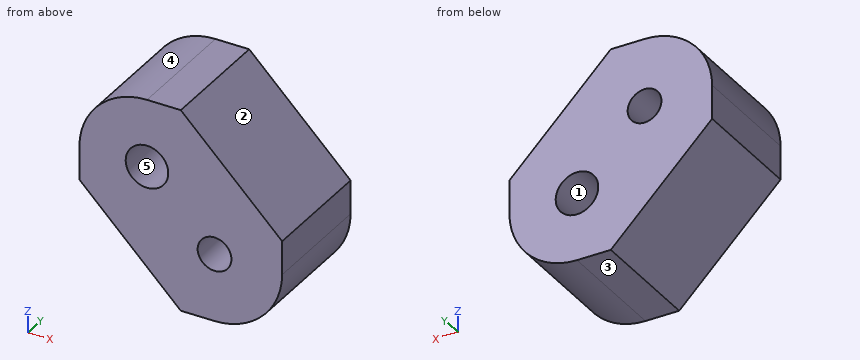
```python
from build123d import *

# Parameters (mm, degrees)
SKETCH1_W           = 19.05
SKETCH1_H           = 19.05
BOSS_EXTRUDE1_DEPTH = 11
SKETCH2_R           = 1.5875
CUT_EXTRUDE1_DEPTH  = 18.39112561
SKETCH3_R           = 2
CUT_EXTRUDE2_DEPTH  = 5.7
SKETCH4_R           = 2
CUT_EXTRUDE3_DEPTH  = 5.7
CUT_EXTRUDE4_DEPTH  = 18.39112561
FILLET1_R           = 6.35


with BuildPart() as part:
    # Sketch1 → Boss-Extrude1 (new body)
    with BuildSketch(Plane(origin=(0, 0, 0), x_dir=(1, 0, 0), z_dir=(0, 1, 0))):
        Rectangle(SKETCH1_W, SKETCH1_H)
    extrude(amount=BOSS_EXTRUDE1_DEPTH)

    # Sketch2 → Cut-Extrude1 (cut, through all)
    with BuildSketch(Plane(origin=(0, 11, 0), x_dir=(1, 0, 0), z_dir=(0, 1, 0))):
        with Locations(Location((-3.175, -3.175, 0), (0, 0, 270))):
            Circle(SKETCH2_R)
        with Locations(Location((3.175, 3.175, 0), (0, 0, 270))):
            Circle(SKETCH2_R)
    extrude(amount=-CUT_EXTRUDE1_DEPTH, mode=Mode.SUBTRACT)

    # Sketch3 → Cut-Extrude2 (cut)
    with BuildSketch(Plane(origin=(0, 11, 0), x_dir=(1, 0, 0), z_dir=(0, 1, 0))):
        with Locations(Location((3.175, 3.175, 0), (0, 0, 270))):
            Circle(SKETCH3_R)
    extrude(amount=-CUT_EXTRUDE2_DEPTH, mode=Mode.SUBTRACT)

    # Sketch4 → Cut-Extrude3 (cut)
    with BuildSketch(Plane.XZ):
        with Locations(Location((-3.175, 3.175, 0), (0, 0, 270))):
            Circle(SKETCH4_R)
    extrude(amount=-CUT_EXTRUDE3_DEPTH, mode=Mode.SUBTRACT)

    # Sketch5 → Cut-Extrude4 (cut, through all)
    with BuildSketch(Plane(origin=(0, 11, 0), x_dir=(1, 0, 0), z_dir=(0, 1, 0))):
        Polygon((-9.525, 9.525), (0, 9.525), (-9.525, 0), align=None)
        Polygon((0, -9.525), (9.525, 0), (9.525, -9.525), align=None)
    extrude(amount=-CUT_EXTRUDE4_DEPTH, mode=Mode.SUBTRACT)

    # Fillet1
    fillet1_edges = [part.edges().sort_by_distance(p)[0] for p in [
        (-9.525, 5.5, 9.525),
        (9.525, 5.5, -9.525),
    ]]
    fillet(fillet1_edges, radius=FILLET1_R)


solid = part.part
```
Part model, mm, in its own coordinate system. Face numbers are marked on the shaded views. A direction names the side the tool comes from. Round coordinates to 2 decimals unless told otherwise and drop trailing zeros. Order: outer loops, then holes, each group sorted by start corner. A loop starts at its lowest first (then second) coordinate and runs counter-clockwise, first axis right, second up. Notation, with made-up numbers: M 3.25,-34.75 L 53.25,-34.75 A15 cw 53.25,-15.75 Z; hole C -19.5,76.25 d3. An arc over 180 degrees is marked long. Put each result on its own line as item: value. Start each with the question number.
1. Slice it at B-B on x = 2.5. List the corners of the cut face in (y, z) (3 decimals), then the cut area to 3 significant figures.
2. Slice it at C-C on z = -2.25. List the corners of the cut face in (x, y) (3 decimals), then the cut area to 3 significant figures.
3. Drop flat-ended pins along their axis: pin 1 (2 mm diameter, centred on x = 2.5, z = -3, fed in from +Y); pin 2 (1 mm diameter, centred on y = 5.5, z = -4, fed in from +X). Give the stop position or say it passes through.
4. Drill centre lines: probe 1 along Z at (x, y) = (-2.75, 9.5) (3 decimals); probe 2 along X at (y, z) = (5.5, 4.5) (3 decimals); probe 3 along X at (y, z) = (2.5, 5) (3 decimals). Where is each one in solid material? Low to high. Write a range as [from, to].
5. Slice it at A-A on y = 4. State how many separate pieces and enclosed holes the cut face has, then the cut area to 3 significant figures.
6. Two-plate mould, pull along Z, no slides. Class the marked faces 1, 2 and 3: +Z half, -Z half, draft (parallel to the pull), parting line (faces both ways), or undercut.
7. Slice it at D-D on x = 6.25. List the corners of the cut face in (y, z) (3 decimals).
8. Tool access for the marked faces 4 and 5: list every direction of +Z, -Z, +X, -X, +Y, -Y with a clear straight run to the whole face (end or side of a thin tool).
Findings:
1. outline: M 0,-9.525 L 11,-9.525 L 11,-5.058 L 5.3,-5.058 L 5.3,-4.612 L 0,-4.612 Z; M 0,-1.738 L 5.3,-1.738 L 5.3,-1.292 L 11,-1.292 L 11,7.025 L 0,7.025 Z
1. area: 145 mm2
2. outline: M -7.275,0 L 1.885,0 L 1.885,5.3 L 1.402,5.3 L 1.402,11 L -7.275,11 Z; M 4.465,0 L 9.525,0 L 9.525,11 L 4.948,11 L 4.948,5.3 L 4.465,5.3 Z
2. area: 151 mm2
3. pin 1: y = 5.3
3. pin 2: x = 9.52
4. probe 1: [-6.775, 1.645], [4.705, 9.525]
4. probe 2: [-9.385, -4.673], [-1.677, 5.025]
4. probe 3: [-9.257, -3.993], [-2.357, 4.525]
5. separate pieces: 1
5. enclosed holes: 2
5. area: 234 mm2
6. face 1: undercut
6. face 2: +Z half
6. face 3: -Z half
7. outline: M 0,-8.731 L 11,-8.731 L 11,3.275 L 0,3.275 Z
8. face 4: +Z, -X, +Y, -Y
8. face 5: -Y
